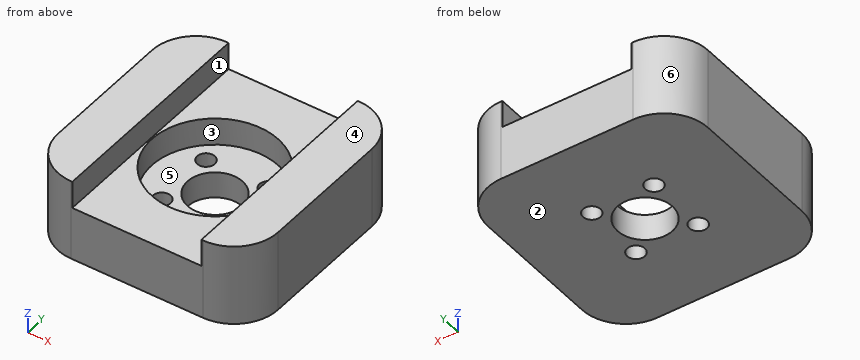
Autodesk Inventor part; units mm, degrees
ref_plane "YZ Plane" through (0, 0, 0) normal (1, 0, 0) x (0, 1, 0)
ref_plane "XZ Plane" through (0, 0, 0) normal (0, 1, 0) x (-1, 0, 0)
ref_plane "XY Plane" through (0, 0, 0) normal (0, 0, 1) x (1, 0, 0)
sketch "Sketch1" plane through (0, 0, 0) normal (0, 1, 0) x (-1, 0, 0)
  line L0 (-20, 7.395) -> (-20, -7.395)
  line L1 (-20, -7.395) -> (20, -7.395)
  line L2 (20, -7.395) -> (20, 7.395)
  line L3 (20, 7.395) -> (11.74, 7.395)
  line L4 (11.74, 7.395) -> (11.74, 2.395)
  line L5 (11.74, 2.395) -> (-11.74, 2.395)
  line L6 (-11.74, 2.395) -> (-11.74, 7.395)
  line L7 (-11.74, 7.395) -> (-20, 7.395)
  point P0 (0, 0)
  point P1 (-20, 0)
  point P2 (-15.87, 7.395)
  point P3 (15.87, 7.395)
  point P4 (0, 2.395)
  dimension "d0" = 40
  dimension "d1" = 14.79
  dimension "d2" = 8.26
  dimension "d3" = 8.26
  dimension "d4" = 5
extrude "Extrusion1" add sketch "Sketch1" along normal mid plane 40
sketch "Sketch2" plane through (-11.74, 20, 2.395) normal (0, 0, 1) x (1, 0, 0)
  circle A0 centre (11.74, -20) radius 11.5
  dimension "d7" = 23
extrude "Extrusion2" cut sketch "Sketch2" against normal blind 5
sketch "Sketch3" plane through (0, 0, -2.605) normal (0, 0, 1) x (1, 0, 0)
  circle A0 centre (0, 0) radius 5
  dimension "d10" = 10
extrude "Extrusion3" cut sketch "Sketch3" against normal up to next
sketch "Sketch4" plane through (0, 0, -2.605) normal (0, 0, 1) x (1, 0, 0)
  circle A0 centre (-5.657, 5.6575) radius 1.6
  circle A1 centre (-5.6575, -5.657) radius 1.6
  circle A2 centre (5.657, -5.6575) radius 1.6
  circle A3 centre (5.6575, 5.657) radius 1.6
  point P0 (0, 0)
  dimension "d13" = 5.657
  dimension "d14" = 5.6575
  dimension "d15" = 3.2
  dimension "d18" = 360
extrude "Extrusion4" cut sketch "Sketch4" against normal up to next
fillet "Fillet1" radius 8 4 edges at (-20, -20, 0) (20, -20, 0) (20, 20, 0) (-20, 20, 0)
properties part number "OldhamCouplerBottom"
Check sheet for the modelled part. Datum: model origin and axes. Units: mm. Face numbers are marked on the shaded views. A direction names the side the tool comes from. Round coordinates to 2 decimals unless told otherwise and drop trailing zeros. Order: outer loops, then holes, each group sorted by start corner. A loop starts at its lowest first (then second) coordinate and runs counter-clockwise, first axis right, second up.
Q1. Cross-section at C-C, the plane y = 0. Enter the section's corners in (x, z) (3 decimals), plus the area to 3 significant figures.
Filled sheet:
outline: (-20, -7.395) - (-5, -7.395) - (-5, -2.605) - (-11.5, -2.605) - (-11.5, 2.395) - (-11.74, 2.395) - (-11.74, 7.395) - (-20, 7.395) - close; (5, -7.395) - (20, -7.395) - (20, 7.395) - (11.74, 7.395) - (11.74, 2.395) - (11.5, 2.395) - (11.5, -2.605) - (5, -2.605) - close
area: 311 mm2
Q2. Cross-section at D-D, the plane z = -2. Enter the section's corners in (x, y), plus the area to 3 significant figures.
Filled sheet:
outline: (-20, -12) arc R8 ccw to (-12, -20) - (12, -20) arc R8 ccw to (20, -12) - (20, 12) arc R8 ccw to (12, 20) - (-12, 20) arc R8 ccw to (-20, 12) - close; hole circle Ø23 at (0, 0)
area: 1,130 mm2
Q3. Scan lines: L1, parallel to X at y = 11, z = 5; L2, parallel to X at y = 7, z = -3.5; L3, parallel to Y at x = 5, z = 0.25. Record each from-to range of solid material in increasing order.
Filled sheet:
L1: x = -20 to -11.74, 11.74 to 20
L2: x = -20 to -6.53, -4.79 to 4.79, 6.53 to 20
L3: y = -20 to -10.36, 10.36 to 20
Q4. Cross-section at A-A, the plane z = 5.5. Enter the section's corners in (x, y).
Filled sheet:
outline: (-20, -12) arc R8 ccw to (-12, -20) - (-11.74, -20) - (-11.74, 20) - (-12, 20) arc R8 ccw to (-20, 12) - close; (11.74, -20) - (12, -20) arc R8 ccw to (20, -12) - (20, 12) arc R8 ccw to (12, 20) - (11.74, 20) - close
Q5. Depth check by flat-ended pin: P1, Ø13, axis at x = 0, y = 0, coming from the -Z side (3 decimals); P2, Ø2.5, axis at x = 5.66, y = 5.66, coming from the -Z side; P3, Ø18.5, axis at x = 0, y = 0, coming from the +Z side (3 decimals). Enter the tip coordinate at first touch or a pass-through.
Filled sheet:
P1: stops at z = -7.395
P2: passes through
P3: stops at z = -2.605
Q6. Set-up check for the marked faces 1, 2 and 3: record each of +Z, -Z, +X, -X, +Y, -Y from which the full face is reachable in a straight line by a thin tool's end or side.
Filled sheet:
face 1: +Z, +Y, -Y
face 2: -Z, +X, -X, +Y, -Y
face 3: +Z
Q7. Draft check along Y on the marked faces 4, 5 and 6. Enter one of: pulls with the +Y half, pulls with the -Y half, needs draft (parallel to the pull), parting line crosses it, or undercut.
Filled sheet:
face 4: needs draft
face 5: undercut
face 6: pulls with the +Y half
Q8. Cross-section at B-B, the plane x = 0. Enter the section's corners in (y, z) (3 decimals), plus the area to 3 significant figures.
Filled sheet:
outline: (-20, -7.395) - (-5, -7.395) - (-5, -2.605) - (-11.5, -2.605) - (-11.5, 2.395) - (-20, 2.395) - close; (5, -7.395) - (20, -7.395) - (20, 2.395) - (11.5, 2.395) - (11.5, -2.605) - (5, -2.605) - close
area: 229 mm2
